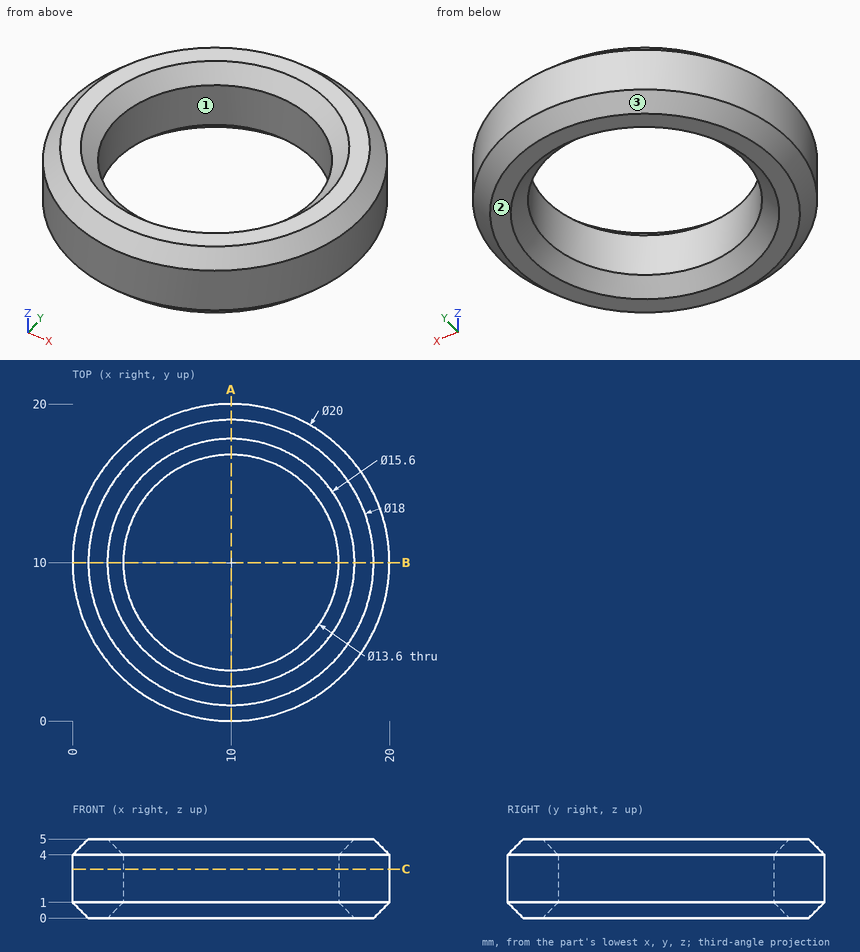
Can you work these out from the drawing? Everything is in mm from the part's minimum corner. Give positions to 0.01 mm unless a question says otherwise; leave off trailing zeros. Order: outer loops, then holes, each group sorted by start corner. A loop starts at its lowest first (then second) coordinate and runs counter-clockwise, first axis right, second up.
1. We'd pull the mould along Y, two halves only. Please class the marked faces 1, 2 and 3: pulls with the +Y half, pulls with the -Y half, needs draft (parallel to the pull), parting line crosses it, or undercut.
2. Suppose I cut it at C-C (z = 3.1). List the corners of the cut face in (x, y) for me.
3. Suppose I cut it at A-A (x = 10). List the corners of the cut face in (y, z) for me, plus the area to 3 significant figures.
4. Will these pins go through, and if not, where does the flat tip stop? P1, Ø1, axis at x = 16, z = 3.5, coming from the -Y side; P2, Ø1, axis at x = 16, z = 4.5, coming from the +Y side; P3, Ø1.5, axis at y = 13.5, z = 2.5, coming from the +X side.
5. I need wall thicknesses on L1, parallel to X at y = 9.75, z = 1.7; L2, parallel to Y at x = 5, z = 3.1. Which ranges of each line are inside material? Lowest first, please.
Solved:
1. face 1: undercut
1. face 2: needs draft
1. face 3: parting line crosses it
2. outline: circle Ø20 at (10, 10); hole circle Ø13.6 at (10, 10)
3. outline: (0, 1) - (1, 0) - (2.2, 0) - (3.2, 1) - (3.2, 4) - (2.2, 5) - (1, 5) - (0, 4) - close; (16.8, 1) - (17.8, 0) - (19, 0) - (20, 1) - (20, 4) - (19, 5) - (17.8, 5) - (16.8, 4) - close
3. area: 28.0 mm2
4. P1: stops at y = 1.65
4. P2: stops at y = 18.1
4. P3: stops at x = 19.61
5. L1: x = 0 to 3.2, 16.8 to 20
5. L2: y = 1.34 to 5.39, 14.61 to 18.66
